The model under review builds one solid part; all positions refer to its coordinate system, in mm. A direction names the side the tool comes from. Give positions to 0.01 mm unless a question says otherwise; leave off trailing zeros. Loops run counter-clockwise (first coordinate to the right, second up) from the corner with the lowest first, then second, coordinate; pieces in that order, holes last. Notation, with made-up numbers: (-35, -30) - (-26, -30) arc R28 cw to (-26, -7) - close; hole circle Ø3 at (-27.5, 66). An arc over 180 degrees is marked (long way). Return JSON: item names as keys, results as strings. Group by question number.
```python
from build123d import *

# Parameters (mm, degrees)
SKETCH1_W           = 57.46
SKETCH1_H           = 23.96
BOSS_EXTRUDE1_DEPTH = 50.2
FILLET1_R           = 1
CUT_EXTRUDE1_REACH  = 25.96
SKETCH2_R           = 3.1
SKETCH2_R_2         = 3
CUT_EXTRUDE2_REACH  = 25.96


with BuildPart() as part:
    # Sketch1 → Boss-Extrude1 (new body)
    with BuildSketch(Plane(origin=(0, 0, 0), x_dir=(0, 0, -1), z_dir=(1, 0, 0))):
        Rectangle(SKETCH1_W, SKETCH1_H)
        with BuildLine():
            Line((-27.5, 1.123993355), (-27.5, 10.75))
            Line((-27.5, 10.75), (27.5, 10.75))
            Line((27.5, 10.75), (27.5, 1.123993355))
            ThreePointArc((27.5, 1.123993355), (26.129235481, 1.667096595), (24.83, 0.97))
            Line((24.83, 0.97), (25.23, 0.67))
            ThreePointArc((25.23, 0.67), (27.48, -0.08), (25.23, -0.83))
            Line((25.23, -0.83), (24.83, -1.13))
            ThreePointArc((24.83, -1.13), (26.129235481, -1.827096595), (27.5, -1.283993355))
            Line((27.5, -1.283993355), (27.5, -3.1))
            Line((27.5, -3.1), (24.3, -3.1))
            Line((24.3, -3.1), (24.3, -3.75))
            Line((24.3, -3.75), (25.3, -3.75))
            Line((25.3, -3.75), (25.3, -6.25))
            Line((25.3, -6.25), (24.3, -6.25))
            Line((24.3, -6.25), (24.3, -6.9))
            Line((24.3, -6.9), (27.5, -6.9))
            Line((27.5, -6.9), (27.5, -10.75))
            Line((27.5, -10.75), (-27.5, -10.75))
            Line((-27.5, -10.75), (-27.5, -6.9))
            Line((-27.5, -6.9), (-24.3, -6.9))
            Line((-24.3, -6.9), (-24.3, -6.25))
            Line((-24.3, -6.25), (-25.3, -6.25))
            Line((-25.3, -6.25), (-25.3, -3.75))
            Line((-25.3, -3.75), (-24.3, -3.75))
            Line((-24.3, -3.75), (-24.3, -3.1))
            Line((-24.3, -3.1), (-27.5, -3.1))
            Line((-27.5, -3.1), (-27.5, -1.283993355))
            ThreePointArc((-27.5, -1.283993355), (-26.129235481, -1.827096595), (-24.83, -1.13))
            Line((-24.83, -1.13), (-25.23, -0.83))
            ThreePointArc((-25.23, -0.83), (-27.48, -0.08), (-25.23, 0.67))
            Line((-25.23, 0.67), (-24.83, 0.97))
            ThreePointArc((-24.83, 0.97), (-26.129235481, 1.667096595), (-27.5, 1.123993355))
        make_face(mode=Mode.SUBTRACT)
    extrude(amount=BOSS_EXTRUDE1_DEPTH)

    # Fillet1
    fillet1_edges = [part.edges().sort_by_distance(p)[0] for p in [
        (25.1, 11.98, -28.73),
        (25.1, -11.98, -28.73),
        (25.1, -11.98, 28.73),
        (25.1, 11.98, 28.73),
    ]]
    fillet(fillet1_edges, radius=FILLET1_R)

    # Sketch2 → Cut-Extrude1 (cut, up to next)
    with BuildSketch(Plane(origin=(0, 11.98, 0), x_dir=(1, 0, 0), z_dir=(0, 1, 0)), mode=Mode.PRIVATE) as cut_extrude1_sk1:
        with Locations((8.25, 18.95)):
            Circle(SKETCH2_R)
        with Locations((8.25, 18.95)):
            Circle(SKETCH2_R_2, mode=Mode.SUBTRACT)
    cut_extrude1_tool1 = extrude(cut_extrude1_sk1.sketch, amount=-CUT_EXTRUDE1_REACH, mode=Mode.PRIVATE) & part.part
    add(cut_extrude1_tool1.solids().sort_by_distance((5.237681, 11.98, -18.95))[0], mode=Mode.SUBTRACT)
    # Sketch2 → Cut-Extrude1 (cut, up to next)
    with BuildSketch(Plane(origin=(0, 11.98, 0), x_dir=(1, 0, 0), z_dir=(0, 1, 0)), mode=Mode.PRIVATE) as cut_extrude1_sk2:
        with Locations((8.25, 18.95)):
            Circle(SKETCH2_R_2)
    cut_extrude1_tool2 = extrude(cut_extrude1_sk2.sketch, amount=-CUT_EXTRUDE1_REACH, mode=Mode.PRIVATE) & part.part
    add(cut_extrude1_tool2.solids().sort_by_distance((8.25, 11.98, -18.95))[0], mode=Mode.SUBTRACT)
    # Sketch2 → Cut-Extrude1 (cut, up to next)
    with BuildSketch(Plane(origin=(0, 11.98, 0), x_dir=(1, 0, 0), z_dir=(0, 1, 0)), mode=Mode.PRIVATE) as cut_extrude1_sk3:
        with Locations((23.55, 18.95)):
            Circle(SKETCH2_R)
        with Locations((23.55, 18.95)):
            Circle(SKETCH2_R_2, mode=Mode.SUBTRACT)
    cut_extrude1_tool3 = extrude(cut_extrude1_sk3.sketch, amount=-CUT_EXTRUDE1_REACH, mode=Mode.PRIVATE) & part.part
    add(cut_extrude1_tool3.solids().sort_by_distance((20.537681, 11.98, -18.95))[0], mode=Mode.SUBTRACT)
    # Sketch2 → Cut-Extrude1 (cut, up to next)
    with BuildSketch(Plane(origin=(0, 11.98, 0), x_dir=(1, 0, 0), z_dir=(0, 1, 0)), mode=Mode.PRIVATE) as cut_extrude1_sk4:
        with Locations((23.55, 18.95)):
            Circle(SKETCH2_R_2)
    cut_extrude1_tool4 = extrude(cut_extrude1_sk4.sketch, amount=-CUT_EXTRUDE1_REACH, mode=Mode.PRIVATE) & part.part
    add(cut_extrude1_tool4.solids().sort_by_distance((23.55, 11.98, -18.95))[0], mode=Mode.SUBTRACT)
    # Sketch2 → Cut-Extrude1 (cut, up to next)
    with BuildSketch(Plane(origin=(0, 11.98, 0), x_dir=(1, 0, 0), z_dir=(0, 1, 0)), mode=Mode.PRIVATE) as cut_extrude1_sk5:
        with Locations((38.85, 18.95)):
            Circle(SKETCH2_R)
        with Locations((38.85, 18.95)):
            Circle(SKETCH2_R_2, mode=Mode.SUBTRACT)
    cut_extrude1_tool5 = extrude(cut_extrude1_sk5.sketch, amount=-CUT_EXTRUDE1_REACH, mode=Mode.PRIVATE) & part.part
    add(cut_extrude1_tool5.solids().sort_by_distance((35.837681, 11.98, -18.95))[0], mode=Mode.SUBTRACT)
    # Sketch2 → Cut-Extrude1 (cut, up to next)
    with BuildSketch(Plane(origin=(0, 11.98, 0), x_dir=(1, 0, 0), z_dir=(0, 1, 0)), mode=Mode.PRIVATE) as cut_extrude1_sk6:
        with Locations((38.85, 18.95)):
            Circle(SKETCH2_R_2)
    cut_extrude1_tool6 = extrude(cut_extrude1_sk6.sketch, amount=-CUT_EXTRUDE1_REACH, mode=Mode.PRIVATE) & part.part
    add(cut_extrude1_tool6.solids().sort_by_distance((38.85, 11.98, -18.95))[0], mode=Mode.SUBTRACT)

    # Sketch3 → Cut-Extrude2 (cut, up to next)
    with BuildSketch(Plane(origin=(0, 11.98, 0), x_dir=(1, 0, 0), z_dir=(0, 1, 0)), mode=Mode.PRIVATE) as cut_extrude2_sk1:
        with BuildLine():
            Line((7.35, 11.35), (7.35, -20.35))
            ThreePointArc((7.35, -20.35), (7.935786438, -21.764213562), (9.35, -22.35))
            Line((9.35, -22.35), (30.75, -22.35))
            ThreePointArc((30.75, -22.35), (32.164213562, -21.764213562), (32.75, -20.35))
            Line((32.75, -20.35), (32.75, 11.35))
            ThreePointArc((32.75, 11.35), (32.164213562, 12.764213562), (30.75, 13.35))
            Line((30.75, 13.35), (9.35, 13.35))
            ThreePointArc((9.35, 13.35), (7.935786438, 12.764213562), (7.35, 11.35))
        make_face()
    cut_extrude2_tool1 = extrude(cut_extrude2_sk1.sketch, amount=-CUT_EXTRUDE2_REACH, mode=Mode.PRIVATE) & part.part
    add(cut_extrude2_tool1.solids().sort_by_distance((20.05, 11.98, 4.5))[0], mode=Mode.SUBTRACT)


solid = part.part
```
1) For pin 1 Ø5.5 at (x, z) = (23.55, -18.95) entering from +Y, flat-tipped, find the tip position at first contact; note if it passes through.
2) Draft analysis for pull direction X (two halves, no side actions). For faces 1 (the face through (0, -11, 2)), 2 (the face through (25, -5, 25.3)), 3 (the face through (7.92, 11.37, 21.75)), state which applies: +X half, -X half, draft (parallel to the pull), parting line (faces both ways), or undercut.
3) We need section D-D, the plane z = -26.23. Write out the cut boundary in (x, y), plus the area to 3 significant figures.
4) To check wall thickness, follow line 1 (Y direction, x = 10.5, z = -26.23); line 2 (Z direction, x = 23.55, y = 11); line 3 (X direction, y = 11.35, z = -18.95). State the ranges of each line that lie inside material, in increasing order.
5) We need section C-C, the plane z = 23. Write out the cut boundary in (x, y), plus the area to 3 significant figures.
6) We need section A-A, the plane z = 6. Write out the cut boundary in (x, y), plus the area to 4 significant figures.
7) Tool access review of faces 4 (the face through (25, 6, -27.5)), 5 (the face through (25, 0, -28.73)), 6 (the face through (35.753, 11.374, -19.086)): name each direction out of +Z, -Z, +X, -X, +Y, -Y from which nothing blocks a thin tool from reaching the whole face with its end or side.
8) We need section B-B, the plane y = -9.5. Write out the cut boundary in (x, z).
Findings:
{
 "1": {"pin 1": "stops at y = -10.75"},
 "2": {"face 1": "-X half", "face 2": "draft", "face 3": "undercut"},
 "3": {"outline": "(0, -11.98) - (50.2, -11.98) - (50.2, -10.75) - (0, -10.75) - close; (0, -6.9) - (50.2, -6.9) - (50.2, -3.1) - (0, -3.1) - close; (0, -1.83) - (50.2, -1.83) - (50.2, -1.33) - (0, -1.33) - close; (0, 1.17) - (50.2, 1.17) - (50.2, 1.67) - (0, 1.67) - close; (0, 10.75) - (50.2, 10.75) - (50.2, 11.98) - (0, 11.98) - close", "area": "364 mm^2"},
 "4": {"line 1": "y = -11.98 to -10.75, -6.9 to -3.1, -1.83 to -1.33, 1.17 to 1.67, 10.75 to 11.98", "line 2": "z = -28.73 to -22.05, -15.85 to -13.35, 22.35 to 28.73", "line 3": "x = 0 to 5.15, 11.35 to 20.45, 26.65 to 35.75, 41.95 to 50.2"},
 "5": {"outline": "(0, -11.98) - (50.2, -11.98) - (50.2, -10.75) - (0, -10.75) - close; (0, 10.75) - (50.2, 10.75) - (50.2, 11.98) - (0, 11.98) - close", "area": "123 mm^2"},
 "6": {"outline": "(0, -11.98) - (50.2, -11.98) - (50.2, -10.75) - (0, -10.75) - close; (0, 10.75) - (7.35, 10.75) - (7.35, 11.98) - (0, 11.98) - close; (32.75, 10.75) - (50.2, 10.75) - (50.2, 11.98) - (32.75, 11.98) - close", "area": "92.25 mm^2"},
 "7": {"face 4": "+X, -X", "face 5": "-Z, +X, -X, +Y, -Y", "face 6": "+Y"},
 "8": {"outline": "(0, -28.73) - (50.2, -28.73) - (50.2, -27.5) - (0, -27.5) - close; (0, 27.5) - (50.2, 27.5) - (50.2, 28.73) - (0, 28.73) - close"}
}
